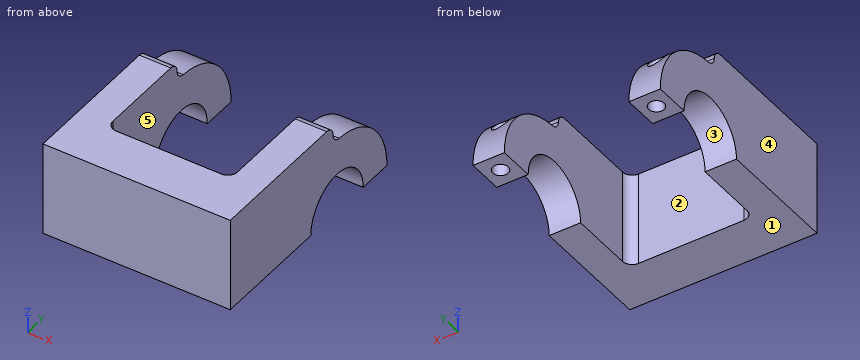
```python
from build123d import *

# Parameters (mm, degrees)
SKETCH3_R            = 15.55
SKETCH3_R_2          = 8.15
BOSS_EXTRUDE4_DEPTH  = 6.5
SKETCH2_R            = 15.55
SKETCH2_R_2          = 8.15
BOSS_EXTRUDE5_DEPTH  = 6.5
CUT_EXTRUDE1_DEPTH   = 38.8
SKETCH5_R            = 1.6
CUT_EXTRUDE2_DEPTH   = 16.55
BOSS_EXTRUDE6_DEPTH  = 6.5
SKETCH9_W            = 6.5
SKETCH9_H            = 21.954006421
BOSS_EXTRUDE7_DEPTH  = 4
BOSS_EXTRUDE8_DEPTH  = 6.5
SKETCH12_W           = 6.5
SKETCH12_H           = 21.954006421
BOSS_EXTRUDE9_DEPTH  = 4
FILLET1_R            = 2
FILLET2_R            = 2
CUT_EXTRUDE3_DEPTH   = 39.8000001
SKETCH13_W           = 19.5
SKETCH13_H           = 10
BOSS_EXTRUDE10_DEPTH = 38.8
FILLET3_R            = 2


with BuildPart() as part:
    # Sketch3 → Boss-Extrude4 (new body)
    with BuildSketch(Plane(origin=(0, 0, 0), x_dir=(0, 0, -1), z_dir=(1, 0, 0))):
        Circle(SKETCH3_R)
        Circle(SKETCH3_R_2, mode=Mode.SUBTRACT)
    extrude(amount=BOSS_EXTRUDE4_DEPTH)


with BuildPart() as body_2:
    # Sketch2 → Boss-Extrude5 (new body)
    with BuildSketch(Plane(origin=(32.3, 0, 0), x_dir=(0, 0, -1), z_dir=(1, 0, 0))):
        Circle(SKETCH2_R)
        Circle(SKETCH2_R_2, mode=Mode.SUBTRACT)
    extrude(amount=BOSS_EXTRUDE5_DEPTH)


with BuildPart() as cut_extrude1_tool:
    # Sketch4 → Cut-Extrude1 (new body)
    with BuildSketch(Plane(origin=(0, 0, 0), x_dir=(0, 0, -1), z_dir=(1, 0, 0))):
        with BuildLine():
            Line((0, 15.55), (0, -15.55))
            ThreePointArc((0, -15.55), (15.55, 0), (0, 15.55))
        make_face()
    extrude(amount=CUT_EXTRUDE1_DEPTH)


with BuildPart() as part_1:
    add(part.part)

    # Cut-Extrude1: cut by cut_extrude1_tool
    add(cut_extrude1_tool.part, mode=Mode.SUBTRACT)


with BuildPart() as body_2_1:
    add(body_2.part)

    # Cut-Extrude1: cut by cut_extrude1_tool
    add(cut_extrude1_tool.part, mode=Mode.SUBTRACT)


with BuildPart() as cut_extrude2_tool:
    # Sketch5 → Cut-Extrude2 (new body, through all)
    with BuildSketch(Plane(origin=(0, 0, 0), x_dir=(-1, 0, 0), z_dir=(0, 0, -1))):
        with Locations((-35.55, 11.85)):
            Circle(SKETCH5_R)
        with Locations((-3.25, 11.85)):
            Circle(SKETCH5_R)
    extrude(amount=-CUT_EXTRUDE2_DEPTH)


with BuildPart() as part_2:
    add(part_1.part)

    # Cut-Extrude2: cut by cut_extrude2_tool
    add(cut_extrude2_tool.part, mode=Mode.SUBTRACT)

    # Sketch11 → Boss-Extrude8 (add)
    with BuildSketch(Plane.ZY):
        with BuildLine():
            ThreePointArc((15.5, -1.245993579), (10.545788255, -11.427547859), (0, -15.55))
            Line((0, -15.55), (0, -23.2))
            Line((0, -23.2), (15.5, -23.2))
            Line((15.5, -23.2), (15.5, -1.245993579))
        make_face()
    extrude(amount=-BOSS_EXTRUDE8_DEPTH)

    # Sketch12 → Boss-Extrude9 (add)
    with BuildSketch(Plane.XY.offset(15.5)):
        with Locations((3.25, -12.22299679)):
            Rectangle(SKETCH12_W, SKETCH12_H)
    extrude(amount=BOSS_EXTRUDE9_DEPTH)

    # Fillet2
    fillet2_edges = [part_2.edges().sort_by_distance(p)[0] for p in [
        (3.25, -1.245993579, 15.5),
    ]]
    fillet(fillet2_edges, radius=FILLET2_R)


with BuildPart() as body_2_2:
    add(body_2_1.part)

    # Cut-Extrude2: cut by cut_extrude2_tool
    add(cut_extrude2_tool.part, mode=Mode.SUBTRACT)

    # Sketch8 → Boss-Extrude6 (add)
    with BuildSketch(Plane(origin=(38.8, 0, 0), x_dir=(0, 0, -1), z_dir=(1, 0, 0))):
        with BuildLine():
            ThreePointArc((0, -19.2), (-8.691551143, -17.120074145), (-15.5, -11.330931118))
            Line((-15.5, -11.330931118), (-15.5, -23.2))
            Line((-15.5, -23.2), (0, -23.2))
            Line((0, -23.2), (0, -19.2))
        make_face()
        with BuildLine():
            ThreePointArc((0, -15.55), (-10.545788255, -11.427547859), (-15.5, -1.245993579))
            Line((-15.5, -1.245993579), (-15.5, -11.330931118))
            ThreePointArc((-15.5, -11.330931118), (-8.691551143, -17.120074145), (0, -19.2))
            Line((0, -19.2), (0, -15.55))
        make_face()
    extrude(amount=-BOSS_EXTRUDE6_DEPTH)

    # Sketch9 → Boss-Extrude7 (add)
    with BuildSketch(Plane.XY.offset(15.5)):
        with Locations((35.55, -12.22299679)):
            Rectangle(SKETCH9_W, SKETCH9_H)
    extrude(amount=BOSS_EXTRUDE7_DEPTH)

    # Fillet1
    fillet1_edges = [body_2_2.edges().sort_by_distance(p)[0] for p in [
        (35.55, -1.245993579, 15.5),
    ]]
    fillet(fillet1_edges, radius=FILLET1_R)


with BuildPart() as cut_extrude3_tool:
    # Sketch10 → Cut-Extrude3 (new body, through all)
    with BuildSketch(Plane(origin=(38.8, 0, 0), x_dir=(0, 0, -1), z_dir=(1, 0, 0))):
        with BuildLine():
            Line((-19.5, -3.212198374), (-19.5, -1.245993579))
            Line((-19.5, -1.245993579), (-17.533795206, -1.245993579))
            ThreePointArc((-17.533795206, -1.245993579), (-18.924111949, -1.82188163), (-19.5, -3.212198374))
        make_face()
    extrude(amount=-CUT_EXTRUDE3_DEPTH)


with BuildPart() as part_3:
    add(part_2.part)

    # Cut-Extrude3: cut by cut_extrude3_tool
    add(cut_extrude3_tool.part, mode=Mode.SUBTRACT)



with BuildPart() as body_2_3:
    add(body_2_2.part)

    # Cut-Extrude3: cut by cut_extrude3_tool
    add(cut_extrude3_tool.part, mode=Mode.SUBTRACT)


with BuildPart() as part_4:
    add(part_3.part)

    add(body_2_3.part)  # Boss-Extrude10 merges body 2
    # Sketch13 → Boss-Extrude10 (add)
    with BuildSketch(Plane(origin=(38.8, 0, 0), x_dir=(0, 0, -1), z_dir=(1, 0, 0))):
        with Locations((-9.75, -28.2)):
            Rectangle(SKETCH13_W, SKETCH13_H)
    extrude(amount=-BOSS_EXTRUDE10_DEPTH)

    # Fillet3
    fillet3_edges = [part_4.edges().sort_by_distance(p)[0] for p in [
        (6.5, -23.2, 9.75),
        (32.3, -23.2, 9.75),
    ]]
    fillet(fillet3_edges, radius=FILLET3_R)


solid = part_4.part
```
Can you work these out from the model? Positions are in its coordinate system, mm. Face numbers are marked on the shaded views. A direction names the side the tool comes from. Coordinates: 2 decimals unless noted, no trailing zeros. Loops run counter-clockwise (first coordinate to the right, second up) from the corner with the lowest first, then second, coordinate; pieces in that order, holes last. Notation, with made-up numbers: M 24.25,35 L 71.25,35 A13 ccw 71.25,55 Z; hole C 18,-27 d10. An arc over 180 degrees is marked long. Put each result on its own line as item: value. Start each with the question number.
(1) Imagine slicing it at A-A on y = -11.5. List the corners of the cut face in (x, z) for me, and give its area (4 significant figures).
(2) Imagine slicing it at C-C on x = 35. List the corners of the cut face in (y, z) for me.
(3) Will these pins go through, and if not, where does the flat tip stop? pin 1 Ø4 at (x, y) = (3.25, 11.85) entering from +Z; pin 2 Ø12 at (x, y) = (25.5, 5.5) entering from +Z.
(4) I need wall thicknesses on probe 1 along X at (y, z) = (11.85, 3.25); probe 2 along X at (y, z) = (-15.5, 18.5); probe 3 along Y at (x, z) = (35.55, 5.75). Which ranges of each line are inside material? Lowest first, please.
(5) Imagine slicing it at B-B on z = 7. List the corners of the cut face in (x, y) for me, and give its area (3 significant figures).
(6) We'd pull the mould along X, two halves only. Please class the marked faces 3, 4 and 5: +X half, -X half, draft (parallel to the pull), parting line (faces both ways), or undercut.
(7) Which directions (+Z, -Z, +X, -X, +Y, -Y) give clear straight access to the entire face, cutting with the end or side of a thin tool? Please do the marked faces 1 and 2.
(8) Imagine slicing it at D-D on y = -5. List the corners of the cut face in (x, z) for me, and give its area (3 significant figures).
Worked answers:
1. outline: M 0,0 L 6.5,0 L 6.5,19.5 L 0,19.5 Z; M 32.3,0 L 38.8,0 L 38.8,19.5 L 32.3,19.5 Z
1. area: 253.5 mm2
2. outline: M -33.2,0 L -8.15,0 A8.15 cw 8.15,0 L 10.35,0 L 10.35,11.61 A15.55 ccw 0.67,15.54 A2 cw -1.25,17.53 A1.97 ccw -3.21,19.5 L -33.2,19.5 Z; M 13.35,0 L 15.55,0 A15.55 ccw 13.35,7.97 Z
3. pin 1: stops at z = 12.03
3. pin 2: passes through
4. probe 1: x = 0 to 1.65, 4.85 to 6.5, 32.3 to 33.95, 37.15 to 38.8
4. probe 2: x = 0 to 6.5, 32.3 to 38.8
4. probe 3: y = -33.2 to -5.78, 5.78 to 10.25, 13.45 to 14.45
5. outline: M 0,-33.2 L 38.8,-33.2 L 38.8,-4.17 L 32.3,-4.17 L 32.3,-21.2 A2 cw 30.3,-23.2 L 8.5,-23.2 A2 cw 6.5,-21.2 L 6.5,-4.17 L 0,-4.17 Z; M 0,4.17 L 6.5,4.17 L 6.5,13.89 L 0,13.89 Z; M 32.3,4.17 L 38.8,4.17 L 38.8,13.89 L 32.3,13.89 Z; hole C 3.25,11.85 d3.2; hole C 35.55,11.85 d3.2
5. area: 747 mm2
6. face 3: draft
6. face 4: -X half
6. face 5: undercut
7. face 1: -Z, +X, -X, +Y, -Y
7. face 2: +Z, -Z, +Y
8. outline: M 0,6.44 L 6.5,6.44 L 6.5,19.5 L 0,19.5 Z; M 32.3,6.44 L 38.8,6.44 L 38.8,19.5 L 32.3,19.5 Z
8. area: 170 mm2
